The listing builds one solid part. Answer for the finished solid, in the listing's coordinates (mm). A direction names the side the tool comes from. Give positions to 0.01 mm unless a question says otherwise; leave off trailing zeros. Write each loop counter-clockwise with the first axis right and the second up, starting at its lowest first coordinate (ties: lowest second). Pieces come first, ordered by that corner, then holes. Notation, with made-up numbers: M -16.75,28 L -8.75,28 A14 cw -8.75,45 Z; hole C -6.75,88 d6. An arc over 180 degrees is marked long. Answer as a JSON object with one key per item and string values.
```python
from build123d import *

# Parameters (mm, degrees)
SKETCH1_W               = 65
SKETCH1_H               = 60
BOSS_EXTRUDE1_DEPTH     = 10
BOSS_EXTRUDE2_DEPTH     = 10
BOSS_EXTRUDE3_START     = -10
BOSS_EXTRUDE3_DEPTH     = 10
CUT_EXTRUDE1_DEPTH      = 101.498756211
CUT_EXTRUDE1_DEPTH_BACK = 101.498756211
SKETCH7_W               = 1.5
SKETCH7_H               = 2
SKETCH7_W_2             = 2
SKETCH7_H_2             = 1.5
SKETCH8_W               = 50
SKETCH8_H               = 3
BOSS_EXTRUDE4_DEPTH     = 20


with BuildPart() as part:
    # Sketch1 → Boss-Extrude1 (new body)
    with BuildSketch(Plane(origin=(0, 0, 0), x_dir=(1, 0, 0), z_dir=(0, 1, 0))):
        with Locations((32.5, 30)):
            Rectangle(SKETCH1_W, SKETCH1_H)
    extrude(amount=BOSS_EXTRUDE1_DEPTH)

    # Sketch2 → Boss-Extrude2 (add)
    with BuildSketch(Plane(origin=(0, 0, -60), x_dir=(-1, 0, 0), z_dir=(0, 0, -1))):
        with BuildLine():
            Line((-65, 10), (-75, 10))
            ThreePointArc((-75, 10), (-80, 5), (-75, 0))
            Line((-75, 0), (-65, 0))
            Line((-65, 0), (-65, 10))
        make_face()
    extrude(amount=-BOSS_EXTRUDE2_DEPTH)

    # Sketch6 → Boss-Extrude3 (add)
    with BuildSketch(Plane.XY.offset(BOSS_EXTRUDE3_START)):
        with BuildLine():
            Line((65, 10), (75, 10))
            ThreePointArc((75, 10), (80, 5), (75, 0))
            Line((75, 0), (65, 0))
            Line((65, 0), (65, 10))
        make_face()
    extrude(amount=BOSS_EXTRUDE3_DEPTH)

    # Sketch7 → Cut-Extrude1 (cut, two sides: drawn at the far end of the back side and taken through both)
    with BuildSketch(Plane.XY.offset(-CUT_EXTRUDE1_DEPTH_BACK)):
        with Locations((76.75, 5)):
            Rectangle(SKETCH7_W, SKETCH7_H)
        with Locations((75, 6.75)):
            Rectangle(SKETCH7_W_2, SKETCH7_H_2)
        with Locations((75, 5)):
            Rectangle(SKETCH7_W_2, SKETCH7_H)
        with Locations((73.25, 5)):
            Rectangle(SKETCH7_W, SKETCH7_H)
        with Locations((75, 3.25)):
            Rectangle(SKETCH7_W_2, SKETCH7_H_2)
    extrude(amount=CUT_EXTRUDE1_DEPTH + CUT_EXTRUDE1_DEPTH_BACK, mode=Mode.SUBTRACT)

    # Sketch8 → Boss-Extrude4 (add)
    with BuildSketch(Plane(origin=(0, 10, 0), x_dir=(1, 0, 0), z_dir=(0, 1, 0))):
        with Locations((32.5, 4.5)):
            Rectangle(SKETCH8_W, SKETCH8_H)
        with Locations((32.5, 55.5)):
            Rectangle(SKETCH8_W, SKETCH8_H)
    extrude(amount=BOSS_EXTRUDE4_DEPTH)


solid = part.part
```
1. A cutting plane is placed at D-D, the plane x = 32.5. Give the vertices of the cut face in (y, z).
Verdict:
{"outline": "M 0,-60 L 10,-60 L 10,-57 L 30,-57 L 30,-54 L 10,-54 L 10,-6 L 30,-6 L 30,-3 L 10,-3 L 10,0 L 0,0 Z"}
2. A cutting plane is placed at B-B, the plane z = -56. Give the vertices of the cut face in (x, y).
Verdict:
{"outline": "M 0,0 L 75,0 A5 ccw 75,10 L 57.5,10 L 57.5,30 L 7.5,30 L 7.5,10 L 0,10 Z; hole M 72.5,4 L 74,4 L 74,2.5 L 76,2.5 L 76,4 L 77.5,4 L 77.5,6 L 76,6 L 76,7.5 L 74,7.5 L 74,6 L 72.5,6 Z"}
3. A cutting plane is placed at C-C, the plane y = 18.5. Give the vertices of the cut face in (x, z).
Verdict:
{"outline": "M 7.5,-57 L 57.5,-57 L 57.5,-54 L 7.5,-54 Z; M 7.5,-6 L 57.5,-6 L 57.5,-3 L 7.5,-3 Z"}
4. Consider line 1 along Z through (x, y) = (56, 16.5); line 2 along Y through (x, z) = (73, -7.5); line 3 along Z through (x, y) = (68.5, 8.5). Determine where each line is inside the solid, lowest interval first.
Verdict:
{"line 1": "z = -57 to -54, -6 to -3", "line 2": "y = 0 to 4, 6 to 10", "line 3": "z = -60 to -50, -10 to 0"}
5. The mould has two halves that part along X. Classify faces 1 (the flat face through (71, 5, -10)), 2 (the flat face through (75, 2.5, -5)), 3 (the flat face through (72.5, 5, -5)), 4 (the cylindrical face through (80, 5, -55)): released by +X, released by -X, zero draft, split by the parting line, or undercut.
Verdict:
{"face 1": "zero draft", "face 2": "undercut", "face 3": "undercut", "face 4": "released by +X"}
6. For faces 5 (the flat face through (77.5, 5, -55)), 6 (the flat face through (65, 5, -30)), 7 (the flat face through (57.5, 20, -4)), determine the directions among +Z, -Z, +X, -X, +Y, -Y from which every point of the face is accessible in a straight line to the end or side of a thin tool.
Verdict:
{"face 5": "+Z, -Z", "face 6": "+X, +Y, -Y", "face 7": "+Z, -Z, +X, +Y"}
7. A cutting plane is placed at A-A, the plane y = 5. Give the vertices of the cut face in (x, z).
Verdict:
{"outline": "M 0,-60 L 72.5,-60 L 72.5,-50 L 65,-50 L 65,-10 L 72.5,-10 L 72.5,0 L 0,0 Z; M 77.5,-60 L 80,-60 L 80,-50 L 77.5,-50 Z; M 77.5,-10 L 80,-10 L 80,0 L 77.5,0 Z"}
8. Flat-ended cylindrical pins translate along their axes: pin 1 (2 mm diameter, centred on x = 10, z = -29.5, fed in from +Y); pin 2 (6 mm diameter, centred on x = 34.5, y = 17, fed in from -Z); pin 3 (4 mm diameter, centred on x = 16, y = 22.5, fed in from +Z). Find the tip coordinate at first contact, or state that the pin passes through.
Verdict:
{"pin 1": "stops at y = 10", "pin 2": "stops at z = -57", "pin 3": "stops at z = -3"}
